```python
from build123d import *

# Parameters (mm, degrees)
SKETCH1_R           = 6
BOSS_EXTRUDE1_DEPTH = 1
SKETCH2_R           = 4
BOSS_EXTRUDE2_DEPTH = 3.5
SKETCH3_R           = 3
CUT_EXTRUDE1_DEPTH  = 11.111874208


with BuildPart() as part:
    # Sketch1 → Boss-Extrude1 (new, symmetric)
    with BuildSketch(Plane(origin=(0, 0, 0), x_dir=(1, 0, 0), z_dir=(0, 1, 0))):
        with Locations(Location((0, 0, 0), (0, 0, 270))):
            Circle(SKETCH1_R)
    extrude(amount=BOSS_EXTRUDE1_DEPTH, both=True)

    # Sketch2 → Boss-Extrude2 (add)
    with BuildSketch(Plane(origin=(0, 1, 0), x_dir=(1, 0, 0), z_dir=(0, 1, 0))):
        with Locations(Location((0, 0, 0), (0, 0, 270))):
            Circle(SKETCH2_R)
    extrude(amount=BOSS_EXTRUDE2_DEPTH)

    # Sketch3 → Cut-Extrude1 (cut, through all)
    with BuildSketch(Plane(origin=(0, 4.5, 0), x_dir=(1, 0, 0), z_dir=(0, 1, 0))):
        with Locations(Location((0, 0, 0), (0, 0, 270))):
            Circle(SKETCH3_R)
    extrude(amount=-CUT_EXTRUDE1_DEPTH, mode=Mode.SUBTRACT)


solid = part.part
```
Work out the finished part from the listing and answer in its coordinate system (mm). A direction names the side the tool comes from. Give positions to 0.01 mm unless a question says otherwise; leave off trailing zeros. Write each loop counter-clockwise with the first axis right and the second up, starting at its lowest first coordinate (ties: lowest second). Pieces come first, ordered by that corner, then holes. Notation, with made-up numbers: (76, 18.25) -> (105, 18.25) arc R17 cw to (105, 34.25) -> close; hole circle Ø9 at (-3.5, 82). An arc over 180 degrees is marked (long way). Write each question's results on one line, items separated by ' | '.
1. Find section C-C on y = -0.5. Determine the outline of the cut face in (x, z), and give its area (3 significant figures).
Data:
outline: circle Ø12 at (0, 0); hole circle Ø6 at (0, 0) | area: 84.8 mm^2
2. Each of these flat-tipped pins is pushed along its axis until it touches: pin 1 Ø5.5 at (x, z) = (0, 0) entering from +Y; pin 2 Ø6 at (x, z) = (-1.5, 0.5) entering from +Y; pin 3 Ø1 at (y, z) = (3.5, 1.5) entering from -X; pin 4 Ø1.5 at (x, y) = (-2, 3) entering from +Z. Where does it stop, or does it pass through?
Data:
pin 1: through | pin 2: y = 4.5 | pin 3: x = -3.87 | pin 4: z = 3.8
3. Straight lines are drawn through the part: L1, parallel to X at y = 0.4, z = 0; L2, parallel to X at y = 1.4, z = 0; L3, parallel to Z at x = -2.25, y = -0.4. For each, find the intervals that lie inside material, in ascending order.
Data:
L1: -6 to -3, 3 to 6 | L2: -4 to -3, 3 to 4 | L3: -5.56 to -1.98, 1.98 to 5.56
4. Find section A-A on x = 0. Determine the outline of the cut face in (y, z), and give its area (3 significant figures).
Data:
outline: (-1, -6) -> (1, -6) -> (1, -4) -> (4.5, -4) -> (4.5, -3) -> (-1, -3) -> close; (-1, 3) -> (4.5, 3) -> (4.5, 4) -> (1, 4) -> (1, 6) -> (-1, 6) -> close | area: 19.0 mm^2
5. Find section B-B on z = 0. Determine the outline of the cut face in (x, y).
Data:
outline: (-6, -1) -> (-3, -1) -> (-3, 4.5) -> (-4, 4.5) -> (-4, 1) -> (-6, 1) -> close; (3, -1) -> (6, -1) -> (6, 1) -> (4, 1) -> (4, 4.5) -> (3, 4.5) -> close
6. Determine the mould class of faces 1 (the cylindrical face through (1.802, 0.014, 5.723)), 2 (the cylindrical face through (0.9, 1.79, 2.86)), 3 (the flat face through (-3.92, 1, -1.42)) for opening direction Z: +Z half, -Z half, draft (parallel to the pull), parting line (faces both ways), or undercut.
Data:
face 1: parting line | face 2: undercut | face 3: draft
7. Find section D-D on z = -3.5. Determine the outline of the cut face in (x, y).
Data:
outline: (-4.87, -1) -> (4.87, -1) -> (4.87, 1) -> (1.94, 1) -> (1.94, 4.5) -> (-1.94, 4.5) -> (-1.94, 1) -> (-4.87, 1) -> close
8. A tool of negligible diameter and unlimited length cuts with its end or side. For faces 4 (the flat face through (3, -1, 1)), 5 (the cylindrical face through (-3.905, 2.726, -0.867)), from which of +Z, -Z, +X, -X, +Y, -Y can it reach the whole face along a straight path? Write none if from no direction.
Data:
face 4: +Z, -Z, +X, -X, -Y | face 5: +Y
